The drawing under review shows one solid part. Ordinate dimensions are in mm from its lowest x, y, z. A direction names the side the tool comes from. Coordinates: 2 decimals unless noted, no trailing zeros. Order: outer loops, then holes, each group sorted by start corner. A loop starts at its lowest first (then second) coordinate and runs counter-clockwise, first axis right, second up.
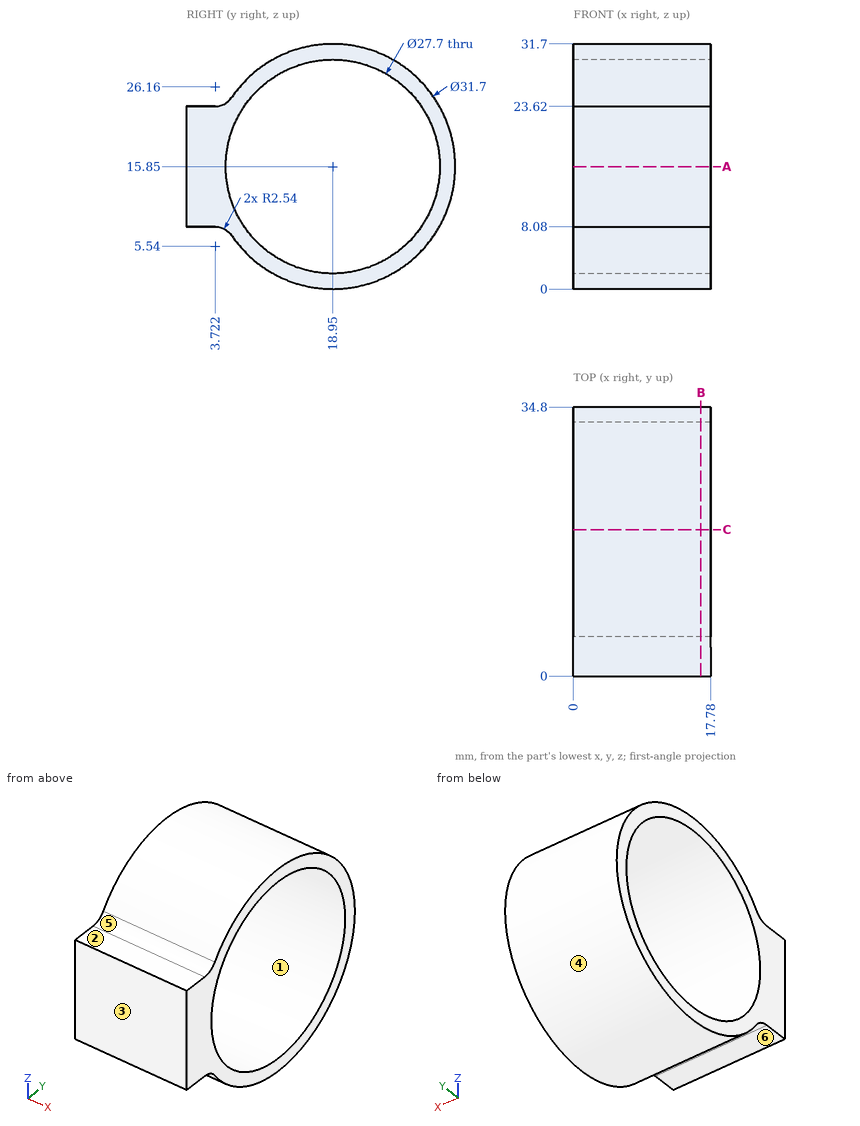
(1) We need section B-B, the plane x = 16.5. Write out the cut boundary in (y, z) (3 decimals), and give its area (3 significant figures).
A:
outline: (0, 8.08) - (3.722, 8.08) arc R2.54 cw to (5.825, 6.964) arc R15.85 ccw (long way) to (5.825, 24.736) arc R2.54 cw to (3.722, 23.62) - (0, 23.62) - close; hole circle Ø27.7 at (18.95, 15.85)
area: 246 mm2
(2) We need section C-C, the plane y = 18.95. Write out the cut boundary in (x, z), and give its area (3 significant figures).
A:
outline: (0, 0) - (17.78, 0) - (17.78, 2) - (0, 2) - close; (0, 29.7) - (17.78, 29.7) - (17.78, 31.7) - (0, 31.7) - close
area: 71.1 mm2
(3) We need section A-A, the plane z = 15.85. Write out the cut boundary in (x, y), and give its area (3 significant figures).
A:
outline: (0, 0) - (17.78, 0) - (17.78, 5.1) - (0, 5.1) - close; (0, 32.8) - (17.78, 32.8) - (17.78, 34.8) - (0, 34.8) - close
area: 126 mm2
(4) Machinability: for the marked faces 5 and 6, which of the approach directions +Z, -Z, +X, -X, +Y, -Y give a long, thin tool a straight path to every point of the face, cutting with its end or side? Answer none if there is none.
A:
face 5: +Z, +X, -X, -Y
face 6: -Z, +X, -X, -Y
(5) For pin 1 Ø4 at (x, y) = (3.5, 4.5) entering from -Z; pin 2 Ø1.1 at (x, y) = (5, 2) entering from +Z; pin 3 Ø8 at (x, y) = (13, 29.5) entering from -Z; pin 4 Ø16.5 at (y, z) = (18.95, 15.85) entering from -X, all flat-tipped, find the tip position at first contact; note any pin that passes through.
A:
pin 1: stops at z = 6.04
pin 2: stops at z = 23.62
pin 3: stops at z = 1.42
pin 4: passes through
(6) Wall thickness on probe 1 along Z at (x, y) = (7.25, 19); probe 2 along Z at (x, y) = (2, 3); probe 3 along Y at (x, z) = (15.75, 6.5): over which ranges is each line inside the solid? List them lowest first.
A:
probe 1: z = 0 to 2, 29.7 to 31.7
probe 2: z = 8.08 to 23.62
probe 3: y = 6.15 to 8.73, 29.17 to 31.75
(7) Draft analysis for pull direction Y (two halves, no side actions). For the marked faces 1, 2, 3 and 4, state which applies: released by +Y, released by -Y, zero draft, split by the parting line, or undercut.
A:
face 1: undercut
face 2: zero draft
face 3: released by -Y
face 4: split by the parting line
